Geometry check sheet. Reference: the model listing, model coordinates, mm. Face numbers are marked on the shaded views. A direction names the side the tool comes from. Give positions to 0.01 mm unless a question says otherwise; leave off trailing zeros. Loops run counter-clockwise (first coordinate to the right, second up) from the corner with the lowest first, then second, coordinate; pieces in that order, holes last. Notation, with made-up numbers: (52.25, -7.75) - (58.25, -7.75) arc R9 cw to (58.25, 5.25) - close; hole circle Ø2 at (42, -0.75). An arc over 180 degrees is marked (long way). Use a Markdown table: item, result. Add a question column.
1. Draft check along Y on the marked faces 1, 2, 3 and 4. Enter one of: pulls with the +Y half, pulls with the -Y half, needs draft (parallel to the pull), parting line crosses it, or undercut.
2. Set-up check for the marked faces 5, 6 and 7: record each of +Z, -Z, +X, -X, +Y, -Y from which the full face is reachable in a straight line by a thin tool's end or side.
3. Cross-section at A-A on x = 124.5. Enter the section's corners in (y, z), and give its area (3 significant figures).
4. Cross-section at B-B on x = 34. Enter the section's corners in (y, z), and give its area (3 significant figures).
5. Material ranges on L1, parallel to X at y = -58.5, z = 22.5; L2, parallel to X at y = 48, z = 20.5; L3, parallel to X at y = 40.5, z = 7.5, recorded low to high.
6. Depth check by flat-ended pin: P1, Ø1, axis at x = 163, y = 50.5, coming from the +Z side; P2, Ø3, axis at x = 184, z = 23.5, coming from the +Y side; P3, Ø9.5, axis at y = 6, z = 17, coming from the -X side. Enter the tip coordinate at first touch or a pass-through.
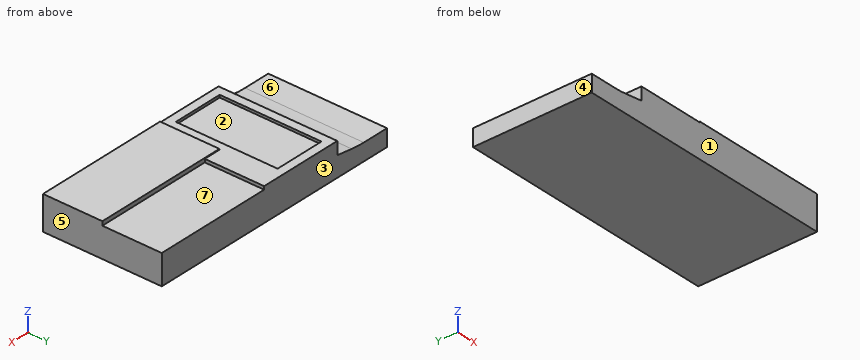
from build123d import *

# Parameters (mm, degrees)
F0_W          = 137.16
F0_H          = 177.8
F1_DEPTH      = 25.4
F3_DEPTH      = 177.801
F4_DEPTH      = 25.4
F5_DEPTH      = 203.2
F7_DEPTH      = 177.801
F8_W          = 88.9
F8_H          = 6.0689005345
F9_DEPTH      = 203.2010001
F10_T4_DEPTH  = 183.39269854
F10_T11_DEPTH = 88.9
F10_T16_DEPTH = 88.9
F11_DEPTH     = 50.8
F12_R         = 152.4
F13_W         = 101.6
F13_H         = 177.8
F14_DEPTH     = 50.8
F15_W         = 76.2
F15_H         = 152.4
F16_DEPTH     = 5.08
F17_DEPTH     = 25.4
F19_DEPTH     = 1.27
F20_DEPTH     = 25.4


# Not quite as in the source:
# - a fillet or chamfer that OpenCascade refuses, or shapes differently, is made with other operations: its cross-section is extruded or revolved along the edge and cut away or added


with BuildPart() as f1:
    # F0 (on Top) → F1 (new body)
    with BuildSketch(Plane.XY):
        Rectangle(F0_W, F0_H)
    extrude(amount=F1_DEPTH)

    # F2 (on face) → F3 (cut, through all)
    with BuildSketch(Plane.XZ.offset(88.9)):
        Polygon((-97.1020311117, 25.4), (-68.58, 0), (68.58, 25.4), (26.2377727777, 59.2203438282), align=None)
    extrude(amount=-F3_DEPTH, mode=Mode.SUBTRACT)

    # F4 (add): a face of the model
    f4_faces = [f1.faces().sort_by_distance(p)[0] for p in [
        (0, 0, 0),
    ]]
    extrude(f4_faces, amount=F4_DEPTH)

    # F5 (add): a face of the model
    f5_faces = [f1.faces().sort_by_distance(p)[0] for p in [
        (68.58, 0, 0),
    ]]
    extrude(f5_faces, amount=F5_DEPTH)

    # F6 (on face) → F7 (cut, through all)
    with BuildSketch(Plane(origin=(0, 88.9, 0), x_dir=(-1, 0, 0), z_dir=(0, 1, 0))):
        with BuildLine():
            add(Edge.make_bspline(
                [(68.58, 0), (45.7187770864, 3.1689187819), (-0.0085622279, 9.5074346586), (-45.7212234372, 16.0563109217), (-68.58, 19.3310994655)],
                knots=[0, 0, 0, 0, 0.4999464928, 1, 1, 1, 1], degree=3))
            Line((68.58, 0), (68.58, 17.6316630095))
            Line((68.58, 17.6316630095), (-68.58, 25.4))
            add(Edge.make_bspline(
                [(-68.58, 19.3310994655), (-68.58, 21.3540663103), (-68.58, 23.3770331552), (-68.58, 25.4)],
                knots=[0, 0, 0, 0, 6.0689005345, 6.0689005345, 6.0689005345, 6.0689005345], degree=3))
        make_face()
    extrude(amount=-F7_DEPTH, mode=Mode.SUBTRACT)

    # F8 (on face) → F9 (cut, through all)
    with BuildSketch(Plane(origin=(68.58, 0, 0), x_dir=(0, -1, 0), z_dir=(-1, 0, 0))):
        with Locations((-44.45, 22.3655497327)):
            Rectangle(F8_W, F8_H)
    extrude(amount=-F9_DEPTH, mode=Mode.SUBTRACT)

    # F10: fillet of radius 127 on 2 edges, made by hand


with BuildPart() as f10_tool2:
    # F10_s3 → F10_t4 (new body)
    with BuildSketch(Plane.XZ.offset(-94.49269854)):
        with BuildLine():
            ThreePointArc((31.1637123625, 13.9794051724), (50.3142381771, 18.2403654673), (68.58, 25.4))
            Line((68.58, 25.4), (69.6868281979, 23.1138391701))
            ThreePointArc((69.6868281979, 23.1138391701), (71.12, 22.3655497327), (71.12, 19.3310994655))
            Line((71.12, 19.3310994655), (68.9402072085, 16.8167703767))
            ThreePointArc((68.9402072085, 16.8167703767), (50.2320909574, 14.1376913402), (31.5222148076, 11.4648324459))
            Line((31.5222148076, 11.4648324459), (31.1637123625, 13.9794051724))
        make_face()
    extrude(amount=F10_T4_DEPTH)

    split(bisect_by=Plane.XZ.offset(-88.9), keep=Keep.TOP)

    split(bisect_by=Plane.XY.offset(19.3310994655), keep=Keep.BOTTOM)

    split(bisect_by=Plane.XZ, keep=Keep.BOTTOM)


with BuildPart() as f1_1:
    add(f1.part)

    # F10_t1: union F10_tool2
    add(f10_tool2.part)


with BuildPart() as f10_tool9:
    # F10_s10 → F10_t11 (new body)
    with BuildSketch(Plane.XZ):
        with BuildLine():
            ThreePointArc((31.1637123625, 13.9794051724), (50.3142381771, 18.2403654673), (68.58, 25.4))
            Line((68.58, 25.4), (69.6868281979, 23.1138391701))
            ThreePointArc((69.6868281979, 23.1138391701), (71.12, 22.3655497327), (71.12, 19.3310994655))
            Line((71.12, 19.3310994655), (68.9402072085, 16.8167703767))
            ThreePointArc((68.9402072085, 16.8167703767), (50.2320909574, 14.1376913402), (31.5222148076, 11.4648324459))
            Line((31.5222148076, 11.4648324459), (31.1637123625, 13.9794051724))
        make_face()
    extrude(amount=F10_T11_DEPTH)

    split(bisect_by=Plane.XY.offset(19.3310994655), keep=Keep.BOTTOM)


with BuildPart() as f1_2:
    add(f1_1.part)

    # F10_t8: union F10_tool9
    add(f10_tool9.part)


with BuildPart() as f10_tool14:
    # F10_s15 → F10_t16 (new body)
    with BuildSketch(Plane.XZ):
        with BuildLine():
            ThreePointArc((31.1637123625, 13.9794051724), (50.3142381771, 18.2403654673), (68.58, 25.4))
            Line((68.58, 25.4), (69.6868281979, 23.1138391701))
            ThreePointArc((69.6868281979, 23.1138391701), (71.12, 22.3655497327), (71.12, 19.3310994655))
            Line((71.12, 19.3310994655), (68.9402072085, 16.8167703767))
            ThreePointArc((68.9402072085, 16.8167703767), (50.2320909574, 14.1376913402), (31.5222148076, 11.4648324459))
            Line((31.5222148076, 11.4648324459), (31.1637123625, 13.9794051724))
        make_face()
    extrude(amount=F10_T16_DEPTH)

    split(bisect_by=Plane.XY.offset(19.3310994655), keep=Keep.TOP)


with BuildPart() as f1_3:
    add(f1_2.part)

    # F10_t13: union F10_tool14
    add(f10_tool14.part)

    # F11 (add): a face of the model
    f11_faces = [f1_3.faces().sort_by_distance(p)[0] for p in [
        (-68.58, 0, -12.7),
    ]]
    extrude(f11_faces, amount=F11_DEPTH)

    # F12
    f12_edges = [f1_3.edges().sort_by_distance(p)[0] for p in [
        (-68.58, 0, 0),
    ]]
    fillet(f12_edges, radius=F12_R)

    # F13 (on face) → F14 (join)
    with BuildSketch(Plane.XY.offset(25.4)):
        with Locations((17.78, 0)):
            Rectangle(F13_W, F13_H)
    extrude(amount=-F14_DEPTH)

    # F15 (on face) → F16 (cut)
    with BuildSketch(Plane.XY.offset(25.4)):
        with Locations((17.78, 0)):
            Rectangle(F15_W, F15_H)
    extrude(amount=-F16_DEPTH, mode=Mode.SUBTRACT)

    # F17 (add): a face of the model
    f17_faces = [f1_3.faces().sort_by_distance(p)[0] for p in [
        (68.58, 44.45, 22.3655497327),
    ]]
    extrude(f17_faces, amount=F17_DEPTH)

    # F18 (on face) → F19 (cut)
    with BuildSketch(Plane.XY.offset(25.4)):
        Polygon((93.98, -88.9), (93.98, 0), (93.98, 88.9), (-33.02, 88.9), (-33.02, -88.9), align=None)
    extrude(amount=-F19_DEPTH, mode=Mode.SUBTRACT)

    # F20 (add): a face of the model
    f20_faces = [f1_3.faces().sort_by_distance(p)[0] for p in [
        (93.98, -44.45, 24.765),
    ]]
    extrude(f20_faces, amount=F20_DEPTH)


solid = f1_3.part
Values found:
| question | item | result |
|---|---|---|
| 1 | face 1 | pulls with the -Y half |
| 1 | face 2 | undercut |
| 1 | face 3 | pulls with the +Y half |
| 1 | face 4 | needs draft |
| 2 | face 5 | +Z, -Z, +X, +Y, -Y |
| 2 | face 6 | +Z, -X, +Y, -Y |
| 2 | face 7 | +Z, +X, +Y |
| 3 | outline | (-88.9, -25.4) - (88.9, -25.4) - (88.9, 19.33) - (0, 19.33) - (0, 25.4) - (-88.9, 25.4) - close |
| 3 | area | 8,490 mm2 |
| 4 | outline | (-88.9, -25.4) - (88.9, -25.4) - (88.9, 24.13) - (76.2, 24.13) - (76.2, 20.32) - (-76.2, 20.32) - (-76.2, 24.13) - (-88.9, 24.13) - close |
| 4 | area | 8,230 mm2 |
| 5 | L1 | x = -33.02 to -20.32, 55.88 to 271.78 |
| 5 | L2 | x = -33.02 to -20.32, 55.88 to 93.98 |
| 5 | L3 | x = -33.02 to 271.78 |
| 6 | P1 | stops at z = 19.33 |
| 6 | P2 | stops at y = 0 |
| 6 | P3 | stops at x = -33.02 |
